Geometry: final body of the model. Coordinates: model frame, mm. Coordinates: 2 decimals unless noted, no trailing zeros. Write each loop counter-clockwise with the first axis right and the second up, starting at its lowest first coordinate (ties: lowest second). Pieces come first, ordered by that corner, then holes. Notation, with made-up numbers: M -12.5,-10.5 L -0.5,-10.5 A37 cw -0.5,26.5 Z; hole C -35,6.5 d11. An arc over 180 degrees is marked long. Write item = value, one per line. Start each with the question number.
Item 1: First-contact query: pin 1 Ø0.9 at (x, z) = (14, 1.5) entering from +Y; pin 2 Ø1 at (y, z) = (-38, 0.5) entering from +X; pin 3 Ø2.5 at (x, y) = (-65, -65) entering from +Z; pin 4 Ø1.5 at (x, z) = (13.5, 2) entering from -Y. Flat tips, straight axial feed; report the tip coordinate or a pass-through.
Item 2: Section C-C on z = 0.5. Give the number of separate pieces and of enclosed holes in the cut face, plus the area to 3 significant figures.
Item 3: Ray query, L1, parallel to Y at x = 25, z = 0.85; L2, parallel to Y at x = -25, z = 1.95; L3, parallel to X at y = -30.5, z = 0.45. Return the intervals inside material, ascending. Write a range as [from, to].
Item 4: Section A-A on x = 18. Output: boundary loops of the cut face in (y, z).
from build123d import *

# Parameters (mm, degrees)
SKETCH_1_W          = 150
SKETCH_1_H          = 150
SKETCH_1_R          = 1.6
EXTRUDE_1_DEPTH     = 3
SKETCH_2_R          = 1.6
CUT_EXTRUDE_1_DEPTH = 3
CUT_EXTRUDE_2_DEPTH = 3


with BuildPart() as part:
    # 草图1 → 凸台-拉伸1 (new body)
    with BuildSketch(Plane.XY):
        Rectangle(SKETCH_1_W, SKETCH_1_H)
        with Locations((-65, 65)):
            Circle(SKETCH_1_R, mode=Mode.SUBTRACT)
        with Locations((65, 65)):
            Circle(SKETCH_1_R, mode=Mode.SUBTRACT)
        with Locations((-65, -65)):
            Circle(SKETCH_1_R, mode=Mode.SUBTRACT)
        with Locations((65, -65)):
            Circle(SKETCH_1_R, mode=Mode.SUBTRACT)
    extrude(amount=EXTRUDE_1_DEPTH)

    # 草图2 → 切除-拉伸1 (cut)
    with BuildSketch(Plane.XY.offset(3)):
        with Locations((-25, -30.505222727)):
            Circle(SKETCH_2_R)
        with Locations((25, -31)):
            Circle(SKETCH_2_R)
        with Locations((25, 31)):
            Circle(SKETCH_2_R)
        with Locations((-25, 31.466039431)):
            Circle(SKETCH_2_R)
        Polygon((75, -55), (75, 55), (60, 40), (60, -40), align=None)
        Polygon((-55, 75), (-40, 60), (40, 60), (55, 75), align=None)
        Polygon((-75, -55), (-60, -40), (-60, 40), (-75, 55), align=None)
        Polygon((-55, -75), (55, -75), (40, -60), (-40, -60), align=None)
    extrude(amount=-CUT_EXTRUDE_1_DEPTH, mode=Mode.SUBTRACT)

    # 草图3 → 切除-拉伸2 (cut)
    with BuildSketch(Plane.XY.offset(3)):
        with BuildLine():
            Line((-5.4, -40.487301924), (-5.4, -37.787301924))
            ThreePointArc((-5.4, -37.787301924), (-5.107106781, -37.080195143), (-4.4, -36.787301924))
            Line((-4.4, -36.787301924), (4.4, -36.787301924))
            ThreePointArc((4.4, -36.787301924), (5.107106781, -37.080195143), (5.4, -37.787301924))
            Line((5.4, -37.787301924), (5.4, -40.487301924))
            ThreePointArc((5.4, -40.487301924), (5.107106781, -41.194408705), (4.4, -41.487301924))
            Line((4.4, -41.487301924), (-4.4, -41.487301924))
            ThreePointArc((-4.4, -41.487301924), (-5.107106781, -41.194408705), (-5.4, -40.487301924))
        make_face()
    extrude(amount=-CUT_EXTRUDE_2_DEPTH, mode=Mode.SUBTRACT)


solid = part.part
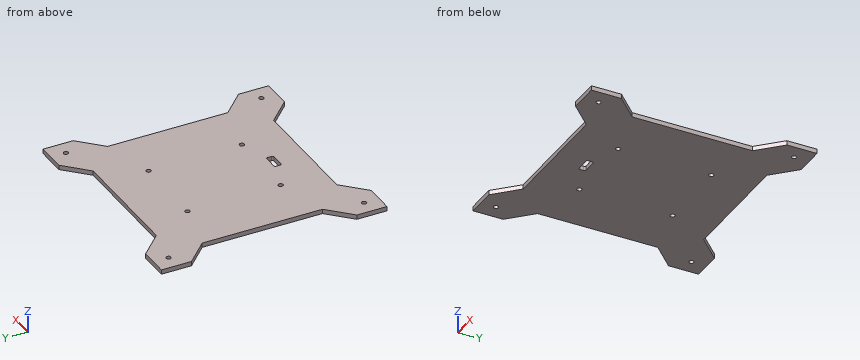
Responses:
q1.pin_1 = 60
q1.pin_2 = 60
q1.pin_3 = through
q1.pin_4 = -60
q2.separate_pieces = 1
q2.enclosed_holes = 9
q2.area = 16,700 mm²
q3.L1 = [-60, -32.6], [-29.4, 29.4], [32.6, 60]
q3.L2 = [-60, -32.11], [-28.91, 29.87], [33.07, 60]
q3.L3 = [-60, -26.6], [-23.4, 23.48], [26.52, 60]
q4.outline = M -60,0 L 60,0 L 60,3 L -60,3 Z
